Autodesk Inventor part; units mm, degrees
ref_plane "YZ Plane" through (0, 0, 0) normal (1, 0, 0) x (0, 1, 0)
ref_plane "XZ Plane" through (0, 0, 0) normal (0, 1, 0) x (-1, 0, 0)
ref_plane "XY Plane" through (0, 0, 0) normal (0, 0, 1) x (1, 0, 0)
sketch "Sketch1" plane through (0, 0, 0) normal (0, 1, 0) x (-1, 0, 0)
  line L0 (0, 0) -> (18, 0)
  line L1 (18, 0) -> (18, -60)
  line L2 (18, -60) -> (0, -60)
  line L3 (0, -60) -> (0, 0)
  dimension "d0" = 18
  dimension "d1" = 60
extrude "Extrusion1" add sketch "Sketch1" along normal blind 1.2
sketch "Sketch3" plane through (-18, 0, 0) normal (0, 0, 1) x (1, 0, 0)
  line L0 (0, 1.2) -> (18, 1.2)
  line L1 (18, 1.2) -> (-52, 1.2)
  line L2 (-52, 1.2) -> (-52, -16.8)
  line L3 (-52, -16.8) -> (18, -16.8)
  line L4 (18, -16.8) -> (18, 1.2)
  point P0 (18, 0)
  dimension "d4" = 70
  dimension "d5" = 18
extrude "Extrusion2" add sketch "Sketch3" along normal blind 1.2
properties part number "Giá đỡ 1"
Geometry check sheet. Reference: the model listing, model coordinates, mm. A direction names the side the tool comes from. Coordinates: 2 decimals unless noted, no trailing zeros. Order: outer loops, then holes, each group sorted by start corner. A loop starts at its lowest first (then second) coordinate and runs counter-clockwise, first axis right, second up.
Q1. Depth check by flat-ended pin: pin 1 Ø5.5 at (x, z) = (-5.5, -27.5) entering from -Y; pin 2 Ø9 at (x, y) = (-20.5, -10.5) entering from -Z. Enter the tip coordinate at first touch or a pass-through.
Reply:
pin 1: stops at y = 0
pin 2: stops at z = 0
Q2. Thickness scan on probe 1 along Y at (x, z) = (-15.5, -45). Record the ranges inside material, lowest first.
Reply:
probe 1: y = 0 to 1.2
Q3. Sectioned sample at C-C on z = -14. Record the cut outline in (x, y), and give its area (3 significant figures).
Reply:
outline: (-18, 0) - (0, 0) - (0, 1.2) - (-18, 1.2) - close
area: 21.6 mm2
Q4. Tool access check on faces 1 (the face through (-12, 1.2, -25)), 2 (the face through (-9, 0, -30)). Record the directions out of +Z, -Z, +X, -X, +Y, -Y that give a thin tool (end or side, any length) a straight path to the whole face; none if there is none.
Reply:
face 1: +Z, -Z, +X, -X, +Y
face 2: -Z, +X, -X, -Y
Q5. Sectioned sample at A-A on x = -8. Record the cut outline in (y, z).
Reply:
outline: (-16.8, 0) - (0, 0) - (0, -60) - (1.2, -60) - (1.2, 1.2) - (-16.8, 1.2) - close
Q6. Sectioned sample at B-B on y = -6.5. Record the cut outline in (x, z).
Reply:
outline: (-70, 0) - (0, 0) - (0, 1.2) - (-70, 1.2) - close
